Answer from the drawing. Dimensions are ordinates in mm from the lowest x, y and z of the part. A direction names the side the tool comes from. Round coordinates to 2 decimals unless told otherwise and drop trailing zeros. Loops run counter-clockwise (first coordinate to the right, second up) from the corner with the lowest first, then second, coordinate; pieces in that order, holes last. Notation, with made-up numbers: M 55.25,-33.75 L 95.25,-33.75 A15 cw 95.25,-19.75 Z; hole C -35.75,-7 d10. An arc over 180 degrees is marked long. One line per item, written item: value.
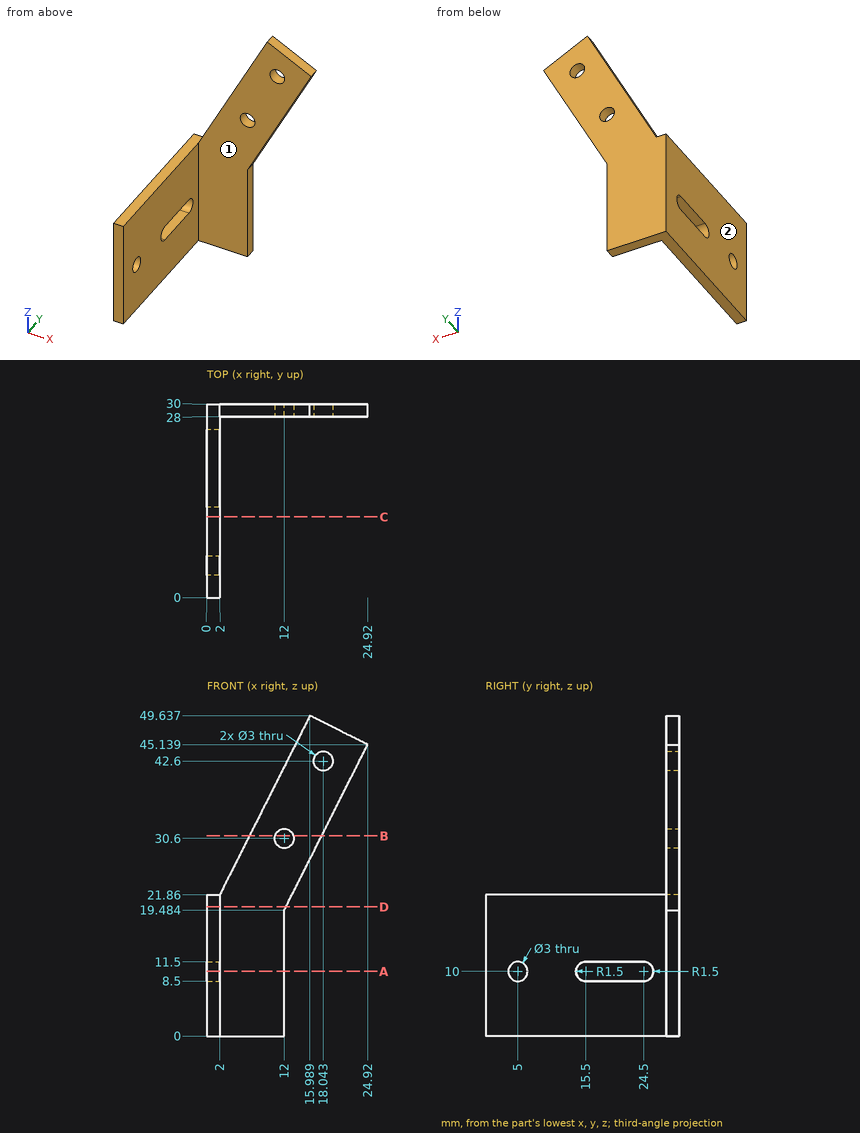
1) Find section D-D (z = 20). Give the vertices of the cut face in (x, y).
Check values:
outline: M 0,0 L 2,0 L 2,28 L 12.26,28 L 12.26,30 L 0,30 Z
2) Find section C-C (y = 12.5). Give the vertices of the cut face in (x, z).
Check values:
outline: M 0,0 L 2,0 L 2,21.86 L 0,21.86 Z
3) Find section A-A (z = 10). Give the vertices of the cut face in (x, y).
Check values:
outline: M 0,0 L 2,0 L 2,3.5 L 0,3.5 Z; M 0,6.5 L 2,6.5 L 2,14 L 0,14 Z; M 0,26 L 2,26 L 2,28 L 12,28 L 12,30 L 0,30 Z
4) Each of these flat-tipped pins is pushed along its axis until it touches: pin 1 (8 mm diameter, centred on x = 14.5, z = 25, fed in from -Y); pin 2 (10 mm diameter, centred on x = 8, y = 5.5, fed in from +Z); pin 3 (1.6 mm diameter, centred on x = 0.5, y = 18.5, fed in from +Z); pin 4 (0.6 mm diameter, centred on y = 29, z = 5, fed in from +X). Where does it stop, or does it pass through?
Check values:
pin 1: y = 28
pin 2: through
pin 3: z = 21.86
pin 4: x = 12
5) Find section B-B (z = 31). Give the vertices of the cut face in (x, y) (1 decimal), then the cut area to 3 significant figures.
Check values:
outline: M 6.6,28 L 10.6,28 L 10.6,30 L 6.6,30 Z; M 13.4,28 L 17.8,28 L 17.8,30 L 13.4,30 Z
area: 16.6 mm2
6) For the marked faces 1 and 2, determine the directions among +Z, -Z, +X, -X, +Y, -Y from which every point of the face is accessible in a straight line to the end or side of a thin tool.
Check values:
face 1: +Z, -Z, +X, -Y
face 2: +Z, -Z, -X, +Y, -Y
7) Find the intervals of material crossed by probe 1 along Z at (x, y) = (1.55, 5); probe 2 along X at (y, z) = (21.25, 8); probe 3 along X at (y, z) = (28.55, 42.6) (1 decimal), in increasing order. Write a range as from..to.
Check values:
probe 1: 0..8.5, 11.5..21.86
probe 2: 0..2
probe 3: 12.4..16.5, 19.5..23.6
